Work out the finished part from the listing and answer in its coordinate system (mm). A direction names the side the tool comes from. Round coordinates to 2 decimals unless told otherwise and drop trailing zeros. Order: outer loops, then holes, each group sorted by start corner. A loop starts at its lowest first (then second) coordinate and runs counter-clockwise, first axis right, second up. Notation, with made-up numbers: (72, -34.75) - (129, -34.75) arc R21 ccw to (129, -12.75) - close; hole circle Ø2 at (-37, -8). An arc over 180 degrees is marked (long way). Answer in a Markdown table with one row per item.
from build123d import *

# Parameters (mm, degrees)
SKETCH1_W           = 18
SKETCH1_H           = 15
BOSS_EXTRUDE1_DEPTH = 3
SKETCH2_W           = 20
SKETCH2_H           = 22
BOSS_EXTRUDE2_DEPTH = 2
SKETCH3_W           = 18.166927201
SKETCH3_H           = 15.903506762
BOSS_EXTRUDE3_DEPTH = 3


with BuildPart() as part:
    # Sketch1 → Boss-Extrude1 (new body)
    with BuildSketch(Plane.XY):
        with Locations((-68.585871194, -139.978474406)):
            Rectangle(SKETCH1_W, SKETCH1_H)
    extrude(amount=BOSS_EXTRUDE1_DEPTH)

    # Sketch2 → Boss-Extrude2 (add)
    with BuildSketch(Plane.XY.offset(3)):
        with Locations((-68.585871194, -142.478474406)):
            Rectangle(SKETCH2_W, SKETCH2_H)
    extrude(amount=BOSS_EXTRUDE2_DEPTH)

    # Sketch3 → Boss-Extrude3 (add)
    with BuildSketch(Plane.XY.offset(5)):
        with Locations((-68.607051799, -144.301260384)):
            Rectangle(SKETCH3_W, SKETCH3_H)
    extrude(amount=BOSS_EXTRUDE3_DEPTH)


solid = part.part
1) Find section B-B, the plane x = -70.25. Give the vertices of the cut face in (y, z), then the cut area to 3 significant figures.
Filled in:
| item | result |
|---|---|
| outline | (-153.48, 3) - (-147.48, 3) - (-147.48, 0) - (-132.48, 0) - (-132.48, 3) - (-131.48, 3) - (-131.48, 5) - (-136.35, 5) - (-136.35, 8) - (-152.25, 8) - (-152.25, 5) - (-153.48, 5) - close |
| area | 137 mm^2 |
2) Find the intervals of material crossed by probe 1 along Z at (x, y) = (-74.25, -151); probe 2 along Z at (x, y) = (-64.75, -135.25); probe 3 along X at (y, z) = (-132.75, 1), in increasing order. Write a range as from..to.
Filled in:
| item | result |
|---|---|
| probe 1 | z = 3..8 |
| probe 2 | z = 0..5 |
| probe 3 | x = -77.59..-59.59 |
3) Find section A-A, the plane y = -151. Give the vertices of the cut face in (x, z), then the cut area to 3 significant figures.
Filled in:
| item | result |
|---|---|
| outline | (-78.59, 3) - (-58.59, 3) - (-58.59, 5) - (-59.52, 5) - (-59.52, 8) - (-77.69, 8) - (-77.69, 5) - (-78.59, 5) - close |
| area | 94.5 mm^2 |
4) Find section D-D, the plane y = -139. Give the vertices of the cut face in (x, z), then the cut area to 3 significant figures.
Filled in:
| item | result |
|---|---|
| outline | (-78.59, 3) - (-77.59, 3) - (-77.59, 0) - (-59.59, 0) - (-59.59, 3) - (-58.59, 3) - (-58.59, 5) - (-59.52, 5) - (-59.52, 8) - (-77.69, 8) - (-77.69, 5) - (-78.59, 5) - close |
| area | 149 mm^2 |
5) Which of the six approach directions +Z, -Z, +X, -X, +Y, -Y give full straight-line access (tool end or side, diameter ignored) to faces 1 (the face through (-77.691, -144, 6)), 2 (the face through (-69, -152.253, 6)), 3 (the face through (-59.524, -144, 6)), 4 (the face through (-69, -136.35, 6))?
Filled in:
| item | result |
|---|---|
| face 1 | +Z, -X, +Y, -Y |
| face 2 | +Z, +X, -X, -Y |
| face 3 | +Z, +X, +Y, -Y |
| face 4 | +Z, +X, -X, +Y |
6) Find section C-C, the plane z = 7.25. Give the vertices of the cut face in (x, y), then the cut area to 3 significant figures.
Filled in:
| item | result |
|---|---|
| outline | (-77.69, -152.25) - (-59.52, -152.25) - (-59.52, -136.35) - (-77.69, -136.35) - close |
| area | 289 mm^2 |
7) Each of these flat-tipped pins is pushed along its axis until it touches: pin 1 (2.5 mm diameter, centred on x = -67, z = 7, fed in from +Y); pin 2 (2.5 mm diameter, centred on x = -71, z = 2, fed in from -Y); pin 3 (1.5 mm diameter, centred on x = -73, z = 6.5, fed in from -Y); pin 4 (1.5 mm diameter, centred on x = -67, z = 1, fed in from +Y). Where does it stop, or does it pass through?
Filled in:
| item | result |
|---|---|
| pin 1 | stops at y = -136.35 |
| pin 2 | stops at y = -153.48 |
| pin 3 | stops at y = -152.25 |
| pin 4 | stops at y = -132.48 |
